Input: dimensioned drawing with shaded views. Units: mm. Origin: part minimum x, y, z. Give positions to 0.01 mm unless a question says otherwise; leave off trailing zeros. Order: outer loops, then holes, each group sorted by start corner. A loop starts at its lowest first (then second) coordinate and runs counter-clockwise, first axis right, second up. Notation, with made-up numbers: M 26.25,-13.5 L 57.25,-13.5 A24 cw 57.25,10.5 Z; hole C 77,48 d1. An arc over 180 degrees is marked long. Answer in a Markdown table with one row per item. Add a question column.
(1) Section query A-A, the plane z = 66. Return loops of the section in (x, y), plus the area to 3 significant figures.
(2) Section query C-C, the plane y = 2.25. Return loops of the section in (x, z), plus the area to 3 significant figures.
(3) Material intervals for line 1 along Y through (x, z) = (5.5, 90); line 2 along X through (y, z) = (20.25, 88.5); line 3 along X through (y, z) = (23.5, 170.5), sorted ascending.
(4) Section query B-B, the plane x = 3.5. Return loops of the section in (y, z) (1 decimal), plus the area to 3 significant figures.
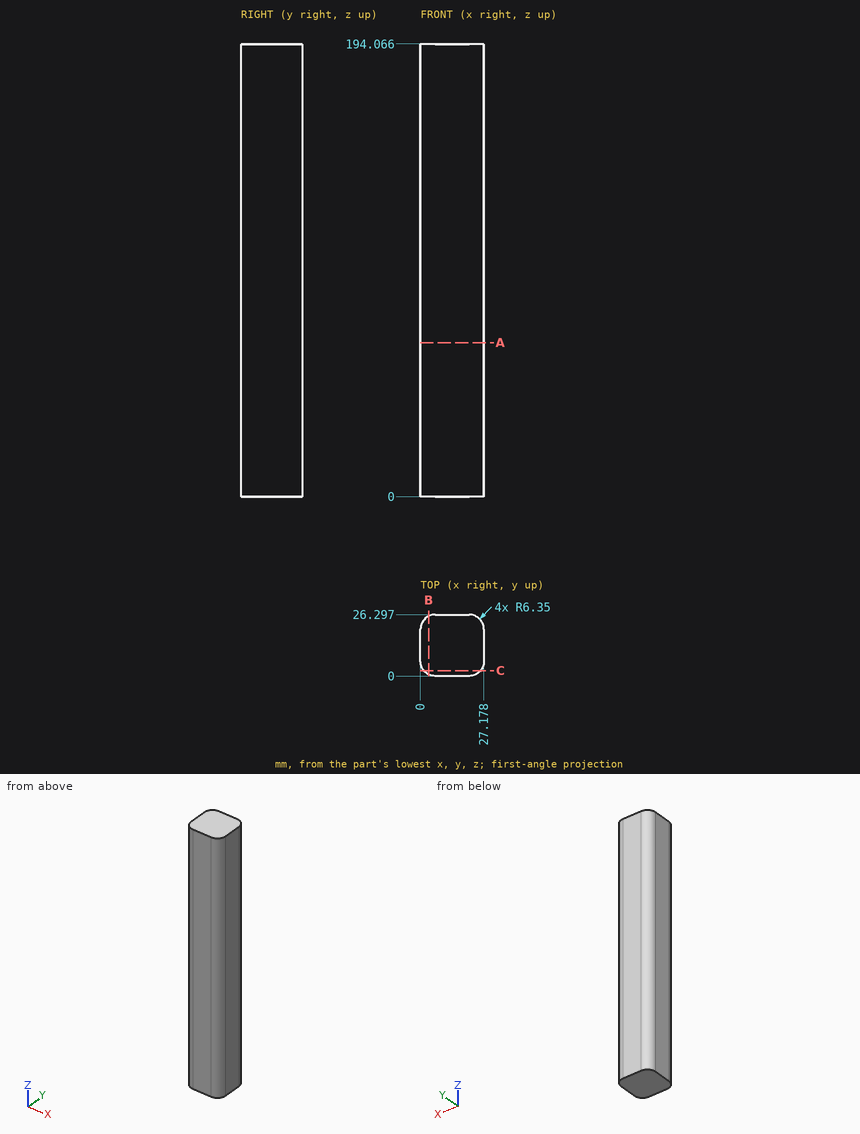
Values follow:
| question | item | result |
|---|---|---|
| 1 | outline | M 0,6.35 A6.35 ccw 6.35,0 L 20.83,0 A6.35 ccw 27.18,6.35 L 27.18,19.95 A6.35 ccw 20.83,26.3 L 6.35,26.3 A6.35 ccw 0,19.95 Z |
| 1 | area | 680 mm² |
| 2 | outline | M 1.5,0 L 25.68,0 L 25.68,194.07 L 1.5,194.07 Z |
| 2 | area | 4,690 mm² |
| 3 | line 1 | y = 0.06 to 26.24 |
| 3 | line 2 | x = 0.01 to 27.17 |
| 3 | line 3 | x = 1.09 to 26.09 |
| 4 | outline | M 0.7,0 L 25.6,0 L 25.6,194.1 L 0.7,194.1 Z |
| 4 | area | 4,840 mm² |
